Can you work these out from the model? Positions are in its coordinate system, mm. Face numbers are marked on the shaded views. Round coordinates to 2 decimals unless told otherwise and drop trailing zeros. Order: outer loops, then holes, each group sorted by start corner. A loop starts at its lowest first (then second) coordinate and runs counter-clockwise, first axis right, second up. Notation, with made-up numbers: M 82,41 L 101,41 A23 ccw 101,52 Z; hole C 71.5,30.5 d1. An arc over 180 degrees is marked long. Answer as CSV lines item,"result". Start each with the question number.
from build123d import *

# Parameters (mm, degrees)
BOSS_EXTRUDE1_DEPTH     = 60
CUT_EXTRUDE1_DEPTH      = 25
CUT_EXTRUDE1_DEPTH_BACK = 25


with BuildPart() as part:
    # Sketch1 → Boss-Extrude1 (new body)
    with BuildSketch(Plane(origin=(0, 0, 0), x_dir=(0, 0, -1), z_dir=(1, 0, 0))):
        Polygon((30.795, 76.26991563), (80.795, -33.73008437), (-30.795, -33.73008437), (-30.795, 76.26991563), align=None)
    extrude(amount=-BOSS_EXTRUDE1_DEPTH)

    # Sketch2 → Cut-Extrude1 (cut, two sides: drawn at the far end of the back side and taken through both)
    with BuildSketch(Plane(origin=(-30, 0, 0), x_dir=(0, 0, -1), z_dir=(1, 0, 0)).offset(-CUT_EXTRUDE1_DEPTH_BACK)):
        Polygon((30.795, 76.26991563), (-25.315, 76.26991563), (-25.315, 71.26991563), (-25.795, 71.26991563), (-25.795, -28.73008437), (78.522272727, -28.73008437), align=None)
    extrude(amount=CUT_EXTRUDE1_DEPTH + CUT_EXTRUDE1_DEPTH_BACK, mode=Mode.SUBTRACT)


solid = part.part
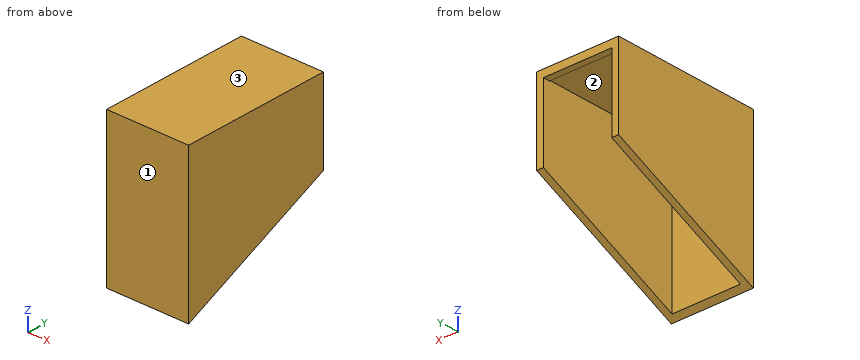
(1) If I drill on line 1 along X through (y, z) = (24.5, -37.5); line 2 along Z through (x, y) = (-47.5, 5) (3 decimals); line 3 along Y through (x, z) = (-44, 5.5), over which ranges is the centre line in solid material (lowest first)?
(2) I'm going to push flat-ended pins straight in: P1, Ø4, axis at x = -26, y = 74.5, coming from the -Z side (3 decimals); P2, Ø10, axis at x = -19.5, y = -3, coming from the -Z side (3 decimals); P3, Ø6, axis at x = -13.5, z = -50.5, coming from the +Y side. Where does each tip first touch, or does it pass through?
(3) I want a section at A-A on x = -49.5. Write out the boundary of the cut face in (y, z) (3 decimals), and give its area (3 significant figures).
(4) If we mould it in two halves opening along Y, with no side actions, what happens to the marked faces 1, 2 and 3? For each: +Y half, -Y half, draft (parallel to the pull), parting line (faces both ways), or undercut.
(5) I want a section at B-B on z = -27.5. Write out the boundary of the cut face in (x, y).
From the geometry:
1,line 1,"-60 to -55, -5 to 0"
1,line 2,"25.795 to 30.795"
1,line 3,"-33.73 to -28.73"
2,P1,"z = 25.315"
2,P2,"z = 25.795"
2,P3,"y = -28.73"
3,outline,"M -33.73,-80.795 L -28.73,-78.522 L -28.73,25.795 L 71.27,25.795 L 71.27,25.315 L 76.27,25.315 L 76.27,30.795 L -33.73,30.795 Z"
3,area,"1,080 mm²"
4,face 1,"-Y half"
4,face 2,"undercut"
4,face 3,"draft"
5,outline,"M -60,-33.73 L 0,-33.73 L 0,76.27 L -5,76.27 L -5,-28.73 L -55,-28.73 L -55,76.27 L -60,76.27 Z"
